Input: part model. Units: mm. Frame: model coordinates. A direction names the side the tool comes from. Give positions to 0.01 mm unless a question says otherwise; leave off trailing zeros. Loops run counter-clockwise (first coordinate to the right, second up) from the corner with the lowest first, then second, coordinate; pieces in that order, holes last. Notation, with made-up numbers: (-35.75, 5.25) -> (-23.75, 5.25) arc R12 ccw to (-23.75, 11.25) -> close; hole circle Ø4 at (6.25, -35.5). An arc over 180 degrees is marked (long way). One line per question, with ' | ' between items.
from build123d import *

# Parameters (mm, degrees)
SKETCH_R     = 1.75
PAD_DEPTH    = 3
SKETCH001_W  = 3
SKETCH001_H  = 63
PAD001_DEPTH = 35
FILLET_R     = 3


with BuildPart() as part:
    # Sketch → Pad (new body)
    with BuildSketch(Plane.XY):
        with BuildLine():
            Line((-81.65, 6), (81.65, 6))
            ThreePointArc((83.15, 4.5), (82.71066, 5.56066), (81.65, 6))
            Line((83.15, 4.5), (83.15, -4.5))
            ThreePointArc((81.65, -6), (82.71066, -5.56066), (83.15, -4.5))
            Line((81.65, -6), (-81.65, -6))
            ThreePointArc((-83.15, -4.5), (-82.71066, -5.56066), (-81.65, -6))
            Line((-83.15, -4.5), (-83.15, 4.5))
            ThreePointArc((-81.65, 6), (-82.71066, 5.56066), (-83.15, 4.5))
        make_face()
        with Locations((-78.65, 0)):
            Circle(SKETCH_R, mode=Mode.SUBTRACT)
        with Locations((78.65, 0)):
            Circle(SKETCH_R, mode=Mode.SUBTRACT)
    extrude(amount=PAD_DEPTH)

    # Sketch001 (on Face11 of Pad) → Pad001 (join)
    with BuildSketch(Plane(origin=(0, 0, 0), x_dir=(1, 0, 0), z_dir=(0, 0, -1))):
        with Locations((12.65, -25.5)):
            Rectangle(SKETCH001_W, SKETCH001_H)
    extrude(amount=-PAD001_DEPTH)

    # Fillet
    fillet_edges = [part.edges().sort_by_distance(p)[0] for p in [
        (12.65, -6, 35),
        (12.65, 57, 35),
        (12.65, 57, 0),
    ]]
    fillet(fillet_edges, radius=FILLET_R)


solid = part.part
1. Ray query, line 1 along Y through (x, z) = (78.65, 1.45); line 2 along X through (y, z) = (20.5, 19); line 3 along Y through (x, z) = (-78, 2). Return the intervals inside material, ascending. Write a range as from..to.
Determined:
line 1: y = -6..-1.75, 1.75..6 | line 2: x = 11.15..14.15 | line 3: y = -6..-1.62, 1.62..6
2. Section query A-A (x = 78.65). Output: boundary loops of the cut face in (y, z).
Determined:
outline: (-6, 0) -> (-1.75, 0) -> (-1.75, 3) -> (-6, 3) -> close; (1.75, 0) -> (6, 0) -> (6, 3) -> (1.75, 3) -> close
3. Section query B-B (x = -14). Output: boundary loops of the cut face in (y, z), then the cut area to 3 significant figures.
Determined:
outline: (-6, 0) -> (6, 0) -> (6, 3) -> (-6, 3) -> close | area: 36.0 mm2
4. Section query C-C (z = 27). Output: boundary loops of the cut face in (x, y), then the cut area to 3 significant figures.
Determined:
outline: (11.15, -6) -> (14.15, -6) -> (14.15, 57) -> (11.15, 57) -> close | area: 189 mm2
5. Pin query (flat end, axial travel): P1, Ø5.5, axis at x = -78.65, y = 0, coming from the +Z side; P2, Ø17.5, axis at y = 17.5, z = 20.5, coming from the -X side; P3, Ø3.5, axis at x = 60, z = 2, coming from the +Y side; P4, Ø3, axis at x = 78.65, y = 0, coming from the -Z side. Return the tip coordinate at first contact, or that it passes through.
Determined:
P1: stops at z = 3 | P2: stops at x = 11.15 | P3: stops at y = 6 | P4: passes through
6. Reachability of faces 1 (the flat face through (49, 0, 3)), 2 (the flat face through (47, 6, 1)), 3 (the flat face through (-35, 0, 3)), 4 (the flat face through (-36, 6, 1)) from +Z, -Z, +X, -X, +Y, -Y: full face, straight path, thin tool, end or side. Return the list, or none.
Determined:
face 1: +Z, +X, +Y, -Y | face 2: +Z, -Z, +X, +Y | face 3: +Z, -X, +Y, -Y | face 4: +Z, -Z, -X, +Y
7. Pull-direction query (X, two-part tool) for faces 5 (the flat face through (13, 57, 17)), 6 (the cylindrical face through (-80.4, 0.08, 1.48)), 7 (the cylindrical face through (76.9, 0.08, 1.48)), 8 (the flat face through (-83.15, 0, 1)); classes: pulls with the +X half, pulls with the -X half, needs draft (parallel to the pull), parting line crosses it, or undercut.
Determined:
face 5: needs draft | face 6: undercut | face 7: undercut | face 8: pulls with the -X half
